```python
from build123d import *

# Parameters (mm, degrees)
F0_W     = 99
F0_H     = 70
F0_R     = 1.1
F0_R_2   = 6.3
F1_DEPTH = 1.5
F2_R     = 5.05
F2_R_2   = 1.1
F2_W     = 59
F2_H     = 10.5
F2_W_2   = 29.5
F2_H_2   = 6
F3_DEPTH = 1.5
F4_R     = 2
F5_R     = 1


with BuildPart() as f1:
    # F0 (on Top) → F1 (new body)
    with BuildSketch(Plane.XY):
        Rectangle(F0_W, F0_H)
        with Locations((-46.5, -26)):
            Circle(F0_R, mode=Mode.SUBTRACT)
        with Locations((-30.5, -26)):
            Circle(F0_R, mode=Mode.SUBTRACT)
        with BuildLine():
            ThreePointArc((-32.5, -14.5), (-32.7928932188, -15.2071067812), (-33.5, -15.5))
            Line((-33.5, -15.5), (-43.5, -15.5))
            ThreePointArc((-43.5, -15.5), (-44.2071067812, -15.2071067812), (-44.5, -14.5))
            Line((-44.5, -14.5), (-44.5, -8.5))
            ThreePointArc((-44.5, -8.5), (-44.2071067812, -7.7928932188), (-43.5, -7.5))
            Line((-43.5, -7.5), (-33.5, -7.5))
            ThreePointArc((-33.5, -7.5), (-32.7928932188, -7.7928932188), (-32.5, -8.5))
            Line((-32.5, -8.5), (-32.5, -14.5))
        make_face(mode=Mode.SUBTRACT)
        with Locations((30.5, -26)):
            Circle(F0_R, mode=Mode.SUBTRACT)
        with Locations((46.5, -26)):
            Circle(F0_R, mode=Mode.SUBTRACT)
        with BuildLine():
            Line((33.5, -7.5), (43.5, -7.5))
            ThreePointArc((43.5, -7.5), (44.2071067812, -7.7928932188), (44.5, -8.5))
            Line((44.5, -8.5), (44.5, -14.5))
            ThreePointArc((44.5, -14.5), (44.2071067812, -15.2071067812), (43.5, -15.5))
            Line((43.5, -15.5), (33.5, -15.5))
            ThreePointArc((33.5, -15.5), (32.7928932188, -15.2071067812), (32.5, -14.5))
            Line((32.5, -14.5), (32.5, -8.5))
            ThreePointArc((32.5, -8.5), (32.7928932188, -7.7928932188), (33.5, -7.5))
        make_face(mode=Mode.SUBTRACT)
        with Locations((-38.5, 3.5)):
            Circle(F0_R_2, mode=Mode.SUBTRACT)
        with Locations((-46.5, 10)):
            Circle(F0_R, mode=Mode.SUBTRACT)
        with Locations((-30.5, 10)):
            Circle(F0_R, mode=Mode.SUBTRACT)
        with Locations((38.5, 3.5)):
            Circle(F0_R_2, mode=Mode.SUBTRACT)
        with Locations((30.5, 10)):
            Circle(F0_R, mode=Mode.SUBTRACT)
        with Locations((46.5, 10)):
            Circle(F0_R, mode=Mode.SUBTRACT)
    extrude(amount=F1_DEPTH)

    # F2 (on face) → F3 (cut, through all)
    with BuildSketch(Plane.XY.offset(1.5)):
        Circle(F2_R)
        with Locations((0, 7)):
            Circle(F2_R_2)
        with Locations((-4.9497474683, 4.9497474683)):
            Circle(F2_R_2)
        with Locations((-7, 0)):
            Circle(F2_R_2)
        with Locations((-4.9497474683, -4.9497474683)):
            Circle(F2_R_2)
        with Locations((0, -7)):
            Circle(F2_R_2)
        with Locations((4.9497474683, -4.9497474683)):
            Circle(F2_R_2)
        with Locations((7, 0)):
            Circle(F2_R_2)
        with Locations((4.9497474683, 4.9497474683)):
            Circle(F2_R_2)
        with BuildLine():
            ThreePointArc((-9.7467943448, 16.8819430161), (-13.3130208521, 19.2849078273), (-17.4008940589, 17.9501778808))
            ThreePointArc((-17.4008940589, 17.9501778808), (-25, 0), (-17.4008940589, -17.9501778808))
            ThreePointArc((-17.4008940589, -17.9501778808), (-13.3130208521, -19.2849078273), (-9.7467943448, -16.8819430161))
            Line((-9.7467943448, -16.8819430161), (-9.643650761, -16.7032930885))
            ThreePointArc((-9.643650761, -16.7032930885), (-9.0333585083, -13.5821275803), (-10.4677200298, -10.7436882577))
            ThreePointArc((-10.4677200298, -10.7436882577), (-15, 0), (-10.4677200298, 10.7436882577))
            ThreePointArc((-10.4677200298, 10.7436882577), (-9.0333585083, 13.5821275803), (-9.643650761, 16.7032930885))
            Line((-9.643650761, 16.7032930885), (-9.7467943448, 16.8819430161))
        make_face()
        with BuildLine():
            ThreePointArc((17.4008940589, 17.9501778808), (13.3130208521, 19.2849078273), (9.7467943448, 16.8819430161))
            Line((9.7467943448, 16.8819430161), (9.643650761, 16.7032930885))
            ThreePointArc((9.643650761, 16.7032930885), (9.0333585083, 13.5821275803), (10.4677200298, 10.7436882577))
            ThreePointArc((10.4677200298, 10.7436882577), (15, 0), (10.4677200298, -10.7436882577))
            ThreePointArc((10.4677200298, -10.7436882577), (9.0333585083, -13.5821275803), (9.643650761, -16.7032930885))
            Line((9.643650761, -16.7032930885), (9.7467943448, -16.8819430161))
            ThreePointArc((9.7467943448, -16.8819430161), (13.3130208521, -19.2849078273), (17.4008940589, -17.9501778808))
            ThreePointArc((17.4008940589, -17.9501778808), (25, 0), (17.4008940589, 17.9501778808))
        make_face()
        with BuildLine():
            Line((-29.5, 35), (-49.5, 35))
            Line((-49.5, 35), (-49.5, 13))
            Line((-49.5, 13), (-31.5, 13))
            ThreePointArc((-31.5, 13), (-30.0857864376, 13.5857864376), (-29.5, 15))
            Line((-29.5, 15), (-29.5, 24.5))
            Line((-29.5, 24.5), (-29.5, 35))
        make_face()
        with Locations((0, 29.75)):
            Rectangle(F2_W, F2_H)
        with BuildLine():
            Line((49.5, 35), (29.5, 35))
            Line((29.5, 35), (29.5, 24.5))
            Line((29.5, 24.5), (29.5, 15))
            ThreePointArc((29.5, 15), (30.0857864376, 13.5857864376), (31.5, 13))
            Line((31.5, 13), (49.5, 13))
            Line((49.5, 13), (49.5, 35))
        make_face()
        Polygon((-20, -35), (20, -35), (20, -29), (20, -24.4319430161), (-20, -24.4319430161), (-20, -29), align=None)
        with Locations((34.75, -32)):
            Rectangle(F2_W_2, F2_H_2)
        with Locations((-34.75, -32)):
            Rectangle(F2_W_2, F2_H_2)
    extrude(amount=-F3_DEPTH, mode=Mode.SUBTRACT)

    # F4
    f4_edges = [f1.edges().sort_by_distance(p)[0] for p in [
        (-20, -24.431943, 0.75),
        (20, -24.431943, 0.75),
    ]]
    fillet(f4_edges, radius=F4_R)

    # F5
    f5_edges = [f1.edges().sort_by_distance(p)[0] for p in [
        (-49.5, -29, 0.75),
        (20, -29, 0.75),
        (-20, -29, 0.75),
        (49.5, -29, 0.75),
        (49.5, 13, 0.75),
        (29.5, 24.5, 0.75),
        (-49.5, 13, 0.75),
        (-29.5, 24.5, 0.75),
    ]]
    fillet(f5_edges, radius=F5_R)


solid = f1.part
```
Work out the finished part from the listing and answer in its coordinate system (mm). Round coordinates to 2 decimals unless told otherwise and drop trailing zeros. Write each loop counter-clockwise with the first axis right and the second up, starting at its lowest first coordinate (ties: lowest second). Pieces come first, ordered by that corner, then holes. Notation, with made-up numbers: (14.25, 48.5) - (61.25, 48.5) arc R19 ccw to (61.25, 52.5) - close; hole circle Ø5 at (53, 48). An arc over 180 degrees is marked (long way). Return JSON: item names as keys, results as strings. Group by question number.
Q1. The part is cut by section A-A on x = -38.5. Write down the section's boundary in (y, z), then the cut area to 3 significant figures.
Q2. The part is cut by section B-B on y = 0. Count the separate pieces of the cut face and the enclosed holes in it, then the cut area to 3 significant figures.
Q3. Find the intervals of material crossed by L1, parallel to Y at x = -46.5, z = 1; L2, parallel to Y at x = -38.5, z = 1.25; L3, parallel to X at y = 8.5, z = 0.35, in increasing order.
Q4. The mould has two halves that part along Y. Classify faces 1 (the flat face through (-1, -14, 1.5)), 2 (the cylindrical face through (0.59, 7.93, 0.76)): released by +Y, released by -Y, zero draft, split by the parting line, or undercut.
Q5. Each of these flat-tipped pins is pushed along its axis until it touches: pin 1 Ø6 at (x, y) = (0, 0) entering from +Z; pin 2 Ø0.8 at (y, z) = (18.5, 0.5) entering from +X. Where does it stop, or does it pass through?
Q6. The part is cut by section C-C on x = 0. Write down the section's boundary in (y, z).
Solved:
{
 "1": {"outline": "(-29, 0) - (-15.5, 0) - (-15.5, 1.5) - (-29, 1.5) - close; (-7.5, 0) - (-2.8, 0) - (-2.8, 1.5) - (-7.5, 1.5) - close; (9.8, 0) - (13, 0) - (13, 1.5) - (9.8, 1.5) - close", "area": "32.1 mm²"},
 "2": {"separate pieces": "8", "enclosed holes": "0", "area": "65.3 mm²"},
 "3": {"L1": "-29 to -27.1, -24.9 to 8.9, 11.1 to 13", "L2": "-29 to -15.5, -7.5 to -2.8, 9.8 to 13", "L3": "-49.5 to -42.33, -34.67 to -23.51, -12.36 to 12.36, 23.51 to 34.67, 42.33 to 49.5"},
 "4": {"face 1": "zero draft", "face 2": "undercut"},
 "5": {"pin 1": "through", "pin 2": "x = 29.5"},
 "6": {"outline": "(-24.43, 0) - (-8.1, 0) - (-8.1, 1.5) - (-24.43, 1.5) - close; (-5.9, 0) - (-5.05, 0) - (-5.05, 1.5) - (-5.9, 1.5) - close; (5.05, 0) - (5.9, 0) - (5.9, 1.5) - (5.05, 1.5) - close; (8.1, 0) - (24.5, 0) - (24.5, 1.5) - (8.1, 1.5) - close"}
}
